Build history of the part. All positions in model axes, mm. Give positions to 0.01 mm unless a question says otherwise; leave off trailing zeros. Order: outer loops, then holes, each group sorted by start corner. A loop starts at its lowest first (then second) coordinate and runs counter-clockwise, first axis right, second up. Notation, with made-up numbers: M 24,-36 L 48,-36 A27 ccw 48,0 Z; hole C 48,-20.75 d8. An arc over 180 degrees is marked long. Answer as CSV lines item,"result".
from build123d import *

# Parameters (mm, degrees)
F1_DEPTH    = 2
F2_R        = 5
F3_R        = 120.7003354098
F4_T1_DEPTH = 5.3985988059
F4_T3_DEPTH = 3.4901996791
F4_T5_DEPTH = 2.6811462233


# Not quite as in the source:
# - a fillet or chamfer that OpenCascade refuses, or shapes differently, is made with other operations: its cross-section is extruded or revolved along the edge and cut away or added
# - a feature names something its author has since deleted; it is built from what else it names


with BuildPart() as f1:
    # F0 (on Right) → F1 (new body)
    with BuildSketch(Plane.YZ):
        with BuildLine():
            add(Edge.make_bspline(
                [(-93.5, -19.165366888), (-87.3498469591, -27.7392359194), (-82.2530835867, -27.7392359194), (-74.081517756, -27.7392359194)],
                knots=[0, 0, 0, 0, 21.227074288, 21.227074288, 21.227074288, 21.227074288], degree=3))
            Line((-74.081517756, -27.7392359194), (-3.9580739103, -27.7392359194))
            Line((-3.9580739103, -27.7392359194), (93.5, -21.748252213))
            Line((93.5, -21.748252213), (147.8121578693, -11.1020449549))
            Line((147.8121578693, -11.1020449549), (168.2493239641, 0))
            Line((168.2493239641, 0), (198.5184252262, 22.1527013928))
            Line((198.5184252262, 22.1527013928), (93.5, 26.4736590703))
            Line((93.5, 26.4736590703), (-2.2493870929, 32.2607640806))
            ThreePointArc((-2.2493870929, 32.2607640806), (-24.7432854958, 19.3285844403), (-47.2371838987, 32.2607640806))
            add(Edge.make_bspline(
                [(-47.2371838987, 32.2607640806), (-62.6581225991, 31.5082555435), (-78.7113010883, 33.5351414979), (-93.5, 30.0032384694)],
                knots=[0, 0, 0, 0, 46.3178645396, 46.3178645396, 46.3178645396, 46.3178645396], degree=3))
            Line((-93.5, 30.0032384694), (-93.5, -19.165366888))
        make_face()
    extrude(amount=F1_DEPTH)

    # F2
    f2_edges = [f1.edges().sort_by_distance(p)[0] for p in [
        (1, -93.5, 30.003238),
        (1, -47.237184, 32.260764),
        (1, -2.249387, 32.260764),
        (1, -93.5, -19.165367),
        (1, -3.958074, -27.739236),
    ]]
    fillet(f2_edges, radius=F2_R)

    # F3
    f3_edges = [f1.edges().sort_by_distance(p)[0] for p in [
        (1, 93.5, -21.748252),
    ]]
    fillet(f3_edges, radius=F3_R)

    # F4: fillet of radius 4.436390167 on 3 edges, made by hand

    # F4_s2 → F4_t1 (cut)
    with BuildSketch(Plane.YZ.offset(-1.699299403)):
        with BuildLine():
            ThreePointArc((147.14513202, -11.2327946013), (147.7946205368, -11.0533364649), (148.4094389633, -10.7775850212))
            Line((148.4094389633, -10.7775850212), (147.8121578693, -11.1020449549))
            Line((147.8121578693, -11.1020449549), (147.14513202, -11.2327946013))
        make_face()
    extrude(amount=F4_T1_DEPTH, mode=Mode.SUBTRACT)

    # F4_s4 → F4_t3 (cut)
    with BuildSketch(Plane.YZ.offset(-0.7450998395)):
        with BuildLine():
            ThreePointArc((167.9874313003, -0.1422674804), (168.2439722622, 0.0084474426), (168.4898338923, 0.176019254))
            Line((168.4898338923, 0.176019254), (168.2493239641, 0))
            Line((168.2493239641, 0), (167.9874313003, -0.1422674804))
        make_face()
    extrude(amount=F4_T3_DEPTH, mode=Mode.SUBTRACT)

    # F4_s6 → F4_t5 (cut)
    with BuildSketch(Plane.YZ.offset(-0.3405731116)):
        with BuildLine():
            ThreePointArc((-3.822101334, -27.730877356), (-3.9581380925, -27.7371457861), (-4.094303155, -27.7392359194))
            Line((-4.094303155, -27.7392359194), (-3.9580739103, -27.7392359194))
            Line((-3.9580739103, -27.7392359194), (-3.822101334, -27.730877356))
        make_face()
    extrude(amount=F4_T5_DEPTH, mode=Mode.SUBTRACT)


solid = f1.part
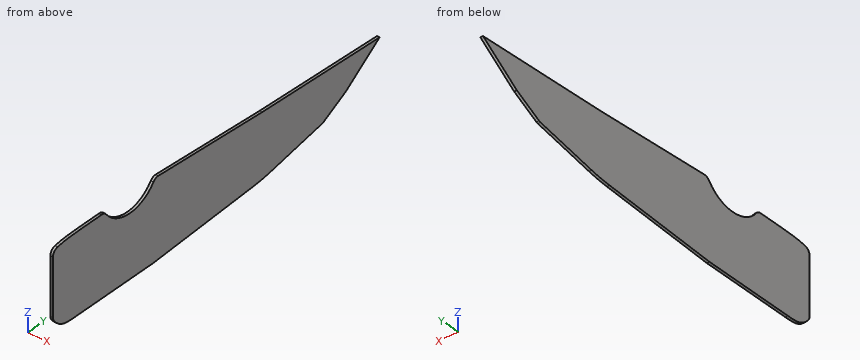
Item 1: Drop a flat-ended pin along its axis: pin 1 (1 mm diameter, centred on x = 0.5, y = -13.5, fed in from +Z). Give the stop position or say it passes through.
Geometry says:
pin 1,"stops at z = 22.13"
Item 2: Band-saw the part on A-A (y = 162.5). Give the cut face in (x, z), and give its area (3 significant figures).
Geometry says:
outline,"M 0,-3.12 L 2,-3.12 L 2,23.63 L 0,23.63 Z"
area,"53.5 mm2"
Item 3: Band-saw the part on B-B (z = 9). Give the cut face in (x, y).
Geometry says:
outline,"M 0,-93.5 L 2,-93.5 L 2,180.55 L 0,180.55 Z"
Item 4: Probe line 1 along Z through (x, y) = (1.45, -59); line 2 along Z through (x, y) = (0.1, -70); line 3 along Y through (x, z) = (1.7, 16). List the from-to ranges inside material, lowest first. Write a range as from..to.
Geometry says:
line 1,"z = -27.74..32.09"
line 2,"z = -27.74..32.18"
line 3,"y = -93.5..190.11"
